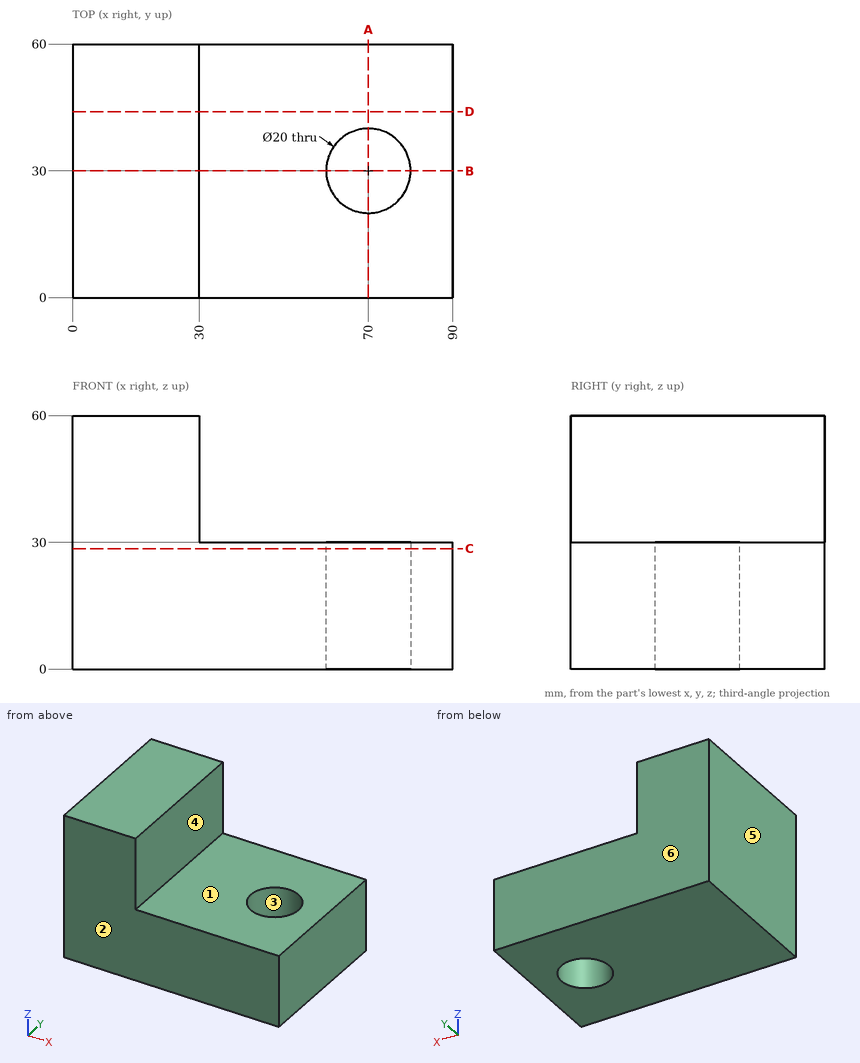
The drawing under review shows one solid part. Ordinate dimensions are in mm from its lowest x, y, z. A direction names the side the tool comes from. Round coordinates to 2 decimals unless told otherwise and drop trailing zeros. Loops run counter-clockwise (first coordinate to the right, second up) from the corner with the lowest first, then second, coordinate; pieces in that order, holes last. Notation, with made-up numbers: (19.5, 83.5) - (54.5, 83.5) arc R30 cw to (54.5, 105.5) - close; hole circle Ø3 at (-3, 68.25). An arc over 180 degrees is marked (long way). Put each result on its own line as item: value. Start each with the question number.
1. For the marked faces 1 and 2, list the 3-axis set-ups (+Z, -Z, +X, -X, +Y, -Y) from which the entire face can be reached by the end or side of a thin tool; tool diameter is ignored.
2. Consider section B-B on y = 30. State the section outline as (x, z) points.
3. Consider section D-D on y = 44. State the section outline as (x, z) points.
4. Consider section A-A on x = 70. State the section outline as (y, z) points, plus the area to 3 significant figures.
5. Insertion check: P1, Ø1, axis at x = 53, y = 26, coming from the +Z side. The pin has a flat end and moves straight along its axis. Give the tip position at first contact, or say it passes through.
6. Consider section C-C on z = 28.5. State the section outline as (x, y) points, plus the area to 3 significant figures.
7. For probe 1 along Y at (x, z) = (70, 13); probe 2 along Z at (x, y) = (44.5, 20.5); probe 3 along X at (y, z) = (38, 14), list the stretches that pass through material, from the lowest coordinate up. Write a range as [from, to].
8. Mouldability with a two-part tool opening along X and no side actions: class the marked faces 3, 4, 5 and 6 as +X half, -X half, draft (parallel to the pull), parting line (faces both ways), or undercut.
Result sheet:
1. face 1: +Z, +X, +Y, -Y
1. face 2: +Z, -Z, +X, -X, -Y
2. outline: (0, 0) - (60, 0) - (60, 30) - (30, 30) - (30, 60) - (0, 60) - close; (80, 0) - (90, 0) - (90, 30) - (80, 30) - close
3. outline: (0, 0) - (90, 0) - (90, 30) - (30, 30) - (30, 60) - (0, 60) - close
4. outline: (0, 0) - (20, 0) - (20, 30) - (0, 30) - close; (40, 0) - (60, 0) - (60, 30) - (40, 30) - close
4. area: 1,200 mm^2
5. P1: z = 30
6. outline: (0, 0) - (90, 0) - (90, 60) - (0, 60) - close; hole circle Ø20 at (70, 30)
6. area: 5,090 mm^2
7. probe 1: [0, 20], [40, 60]
7. probe 2: [0, 30]
7. probe 3: [0, 64], [76, 90]
8. face 3: undercut
8. face 4: +X half
8. face 5: -X half
8. face 6: draft
